Here's the drawing with two shaded views (mm, measured from the low corner). I have some questions. Coordinates: 2 decimals unless noted, no trailing zeros. Loops run counter-clockwise (first coordinate to the right, second up) from the corner with the lowest first, then second, coordinate; pieces in that order, holes last. Notation, with made-up numbers: (88, -0.75) -> (97, -0.75) arc R19 ccw to (97, 11.25) -> close; hole circle Ø4 at (-24, -17). An arc over 180 degrees is marked (long way). Answer as a JSON object with one key per item and string values. Group by question number.
Q1. I want a section at C-C on y = 5. Write out the boundary of the cut face in (x, z), then the cut area to 3 significant figures.
Q2. I want a section at D-D on y = 7.25. Write out the boundary of the cut face in (x, z), then the cut area to 3 significant figures.
Q3. I want a section at A-A on x = 2.5. Write out the boundary of the cut face in (y, z).
Q4. I need wall thicknesses on line 1 (Y direction, x = 2.5, z = 1.95); line 2 (X direction, y = 3, z = 2.15); line 3 (X direction, y = 3.5, z = 1). Which ranges of each line are inside material? Lowest first, please.
Q5. Thinking about a two-plate mould opening in X: for the marked faces 1, 2, 3 and 4, which applies, released by +X, released by -X, zero draft, split by the parting line, or undercut?
Q6. I want a section at B-B on z = 1.3. Write out the boundary of the cut face in (x, y), then the cut area to 3 significant figures.
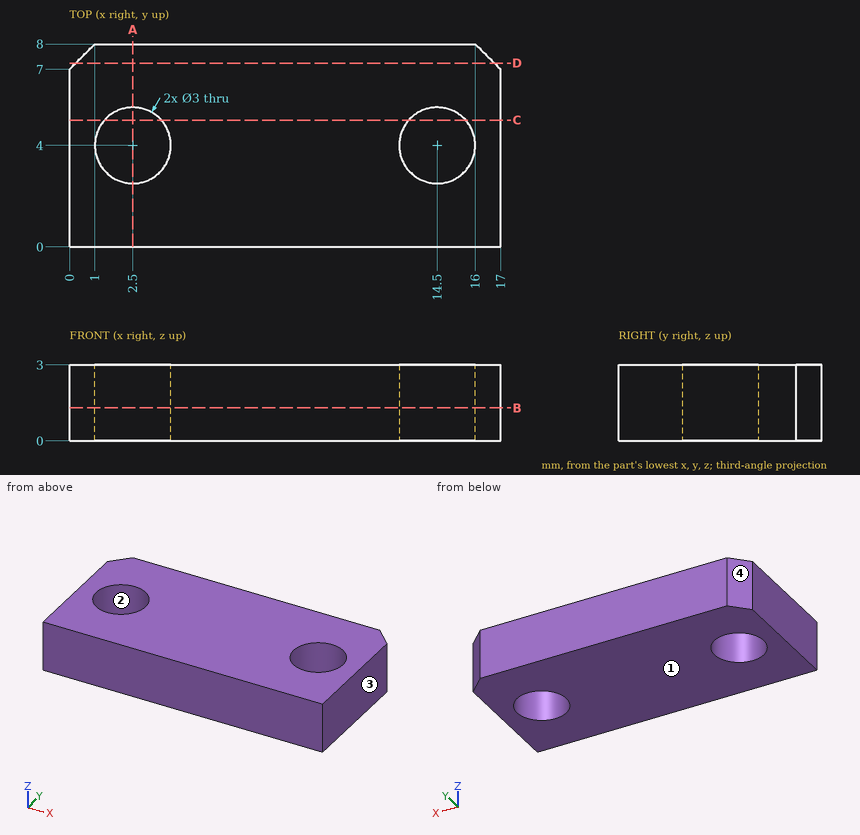
Result set:
{
 "1": {"outline": "(0, 0) -> (1.38, 0) -> (1.38, 3) -> (0, 3) -> close; (3.62, 0) -> (13.38, 0) -> (13.38, 3) -> (3.62, 3) -> close; (15.62, 0) -> (17, 0) -> (17, 3) -> (15.62, 3) -> close", "area": "37.6 mm²"},
 "2": {"outline": "(0.25, 0) -> (16.75, 0) -> (16.75, 3) -> (0.25, 3) -> close", "area": "49.5 mm²"},
 "3": {"outline": "(0, 0) -> (2.5, 0) -> (2.5, 3) -> (0, 3) -> close; (5.5, 0) -> (8, 0) -> (8, 3) -> (5.5, 3) -> close"},
 "4": {"line 1": "y = 0 to 2.5, 5.5 to 8", "line 2": "x = 0 to 1.38, 3.62 to 13.38, 15.62 to 17", "line 3": "x = 0 to 1.09, 3.91 to 13.09, 15.91 to 17"},
 "5": {"face 1": "zero draft", "face 2": "undercut", "face 3": "released by +X", "face 4": "released by -X"},
 "6": {"outline": "(0, 0) -> (17, 0) -> (17, 7) -> (16, 8) -> (1, 8) -> (0, 7) -> close; hole circle Ø3 at (2.5, 4); hole circle Ø3 at (14.5, 4)", "area": "121 mm²"}
}
